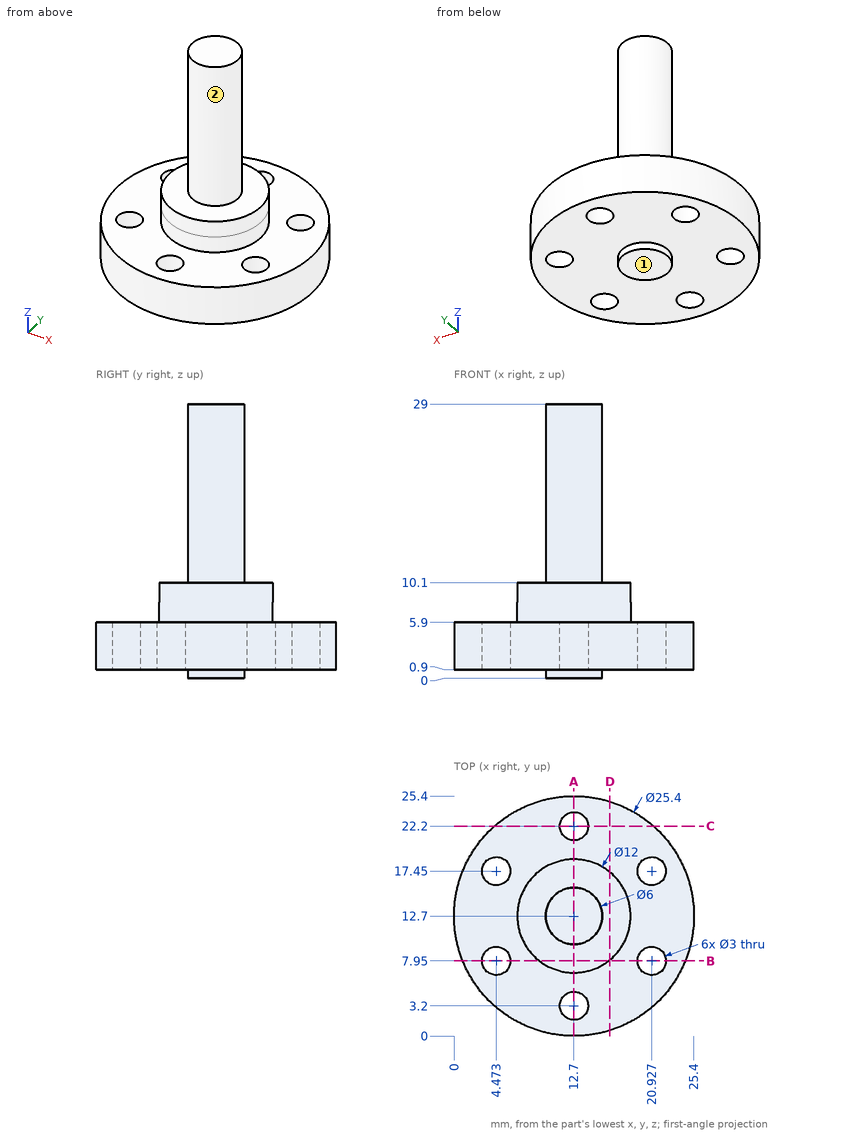
Design review of the part shown in the three views and the two pictorial views. Dimensions are in mm from the part's minimum x, y and z. A direction names the side the tool comes from. Give positions to 0.01 mm unless a question says otherwise; leave off trailing zeros. Loops run counter-clockwise (first coordinate to the right, second up) from the corner with the lowest first, then second, coordinate; pieces in that order, holes last. Notation, with made-up numbers: (-3.5, 6.5) -> (40.5, 6.5) arc R22 cw to (40.5, 36.5) -> close; hole circle Ø8 at (-11, 49.25). An arc over 180 degrees is marked (long way). Answer as a JSON object with one key per item and string values. Group by question number.
Q1. Take a section at D-D (x = 16.5). Write out the cut boundary in (y, z), plus the area to 3 significant figures.
Q2. Insertion check: pin 1 (2 mm diameter, centred on x = 11, z = 21, fed in from +Y); pin 2 (8 mm diameter, centred on x = 9.5, z = 4, fed in from +Y); pin 3 (10 mm diameter, centred on x = 12.5, z = 17.5, fed in from +Y); pin 4 (1 mm diameter, centred on y = 9, z = 10, fed in from +X) (1 decimal). Each pin has a flat end and moves straight along its axis. Give the tip position at first contact, or say it passes through.
Q3. Take a section at A-A (x = 12.7). Write out the cut boundary in (y, z), plus the area to 3 significant figures.
Q4. Take a section at C-C (y = 22.2). Write out the cut boundary in (x, z), plus the area to 3 significant figures.
Q5. Tool access review of the marked faces 1 and 2: name each direction out of +Z, -Z, +X, -X, +Y, -Y from which nothing blocks a thin tool from reaching the whole face with its end or side.
Q6. Take a section at B-B (y = 7.95). Write out the cut boundary in (x, z), plus the area to 3 significant figures.
Q7. Wall thickness on line 1 along Z through (x, y) = (17.5, 18); line 2 along Y through (x, z) = (11.75, 23.75) (1 decimal); line 3 along X through (y, z) = (15, 3.25): over which ranges is each line inside the solid? List them lowest first.
Answer below:
{
 "1": {"outline": "(0.58, 0.9) -> (24.82, 0.9) -> (24.82, 5.9) -> (17.34, 5.9) -> (17.34, 10.1) -> (8.06, 10.1) -> (8.06, 5.9) -> (0.58, 5.9) -> close", "area": "160 mm2"},
 "2": {"pin 1": "stops at y = 15.62", "pin 2": "stops at y = 25.4", "pin 3": "stops at y = 15.7", "pin 4": "stops at x = 17.8"},
 "3": {"outline": "(0, 0.9) -> (1.7, 0.9) -> (1.7, 5.9) -> (0, 5.9) -> close; (4.7, 0.9) -> (9.7, 0.9) -> (9.7, 0) -> (15.7, 0) -> (15.7, 0.9) -> (20.7, 0.9) -> (20.7, 5.9) -> (18.7, 5.9) -> (18.7, 10.1) -> (15.7, 10.1) -> (15.7, 29) -> (9.7, 29) -> (9.7, 10.1) -> (6.7, 10.1) -> (6.7, 5.9) -> (4.7, 5.9) -> close; (23.7, 0.9) -> (25.4, 0.9) -> (25.4, 5.9) -> (23.7, 5.9) -> close", "area": "266 mm2"},
 "4": {"outline": "(4.27, 0.9) -> (11.2, 0.9) -> (11.2, 5.9) -> (4.27, 5.9) -> close; (14.2, 0.9) -> (21.13, 0.9) -> (21.13, 5.9) -> (14.2, 5.9) -> close", "area": "69.3 mm2"},
 "5": {"face 1": "-Z, +X, -X, +Y, -Y", "face 2": "+Z"},
 "6": {"outline": "(0.92, 0.9) -> (2.97, 0.9) -> (2.97, 5.9) -> (0.92, 5.9) -> close; (5.97, 0.9) -> (19.43, 0.9) -> (19.43, 5.9) -> (16.37, 5.9) -> (16.37, 10.1) -> (9.03, 10.1) -> (9.03, 5.9) -> (5.97, 5.9) -> close; (22.43, 0.9) -> (24.48, 0.9) -> (24.48, 5.9) -> (22.43, 5.9) -> close", "area": "119 mm2"},
 "7": {"line 1": "z = 0.9 to 5.9", "line 2": "y = 9.9 to 15.5", "line 3": "x = 0.21 to 25.19"}
}
